Verification items for this drawing (mm, ordinates from the low corner). A direction names the side the tool comes from. Coordinates: 2 decimals unless noted, no trailing zeros. Order: outer loops, then holes, each group sorted by start corner. A loop starts at its lowest first (then second) coordinate and runs counter-clockwise, first axis right, second up. Notation, with made-up numbers: (6, 84.25) -> (47, 84.25) arc R28 cw to (47, 108.25) -> close; hole circle Ø7 at (-39.75, 10.5). An arc over 180 degrees is marked (long way). Answer as CSV lines item,"result". Start each with the question number.
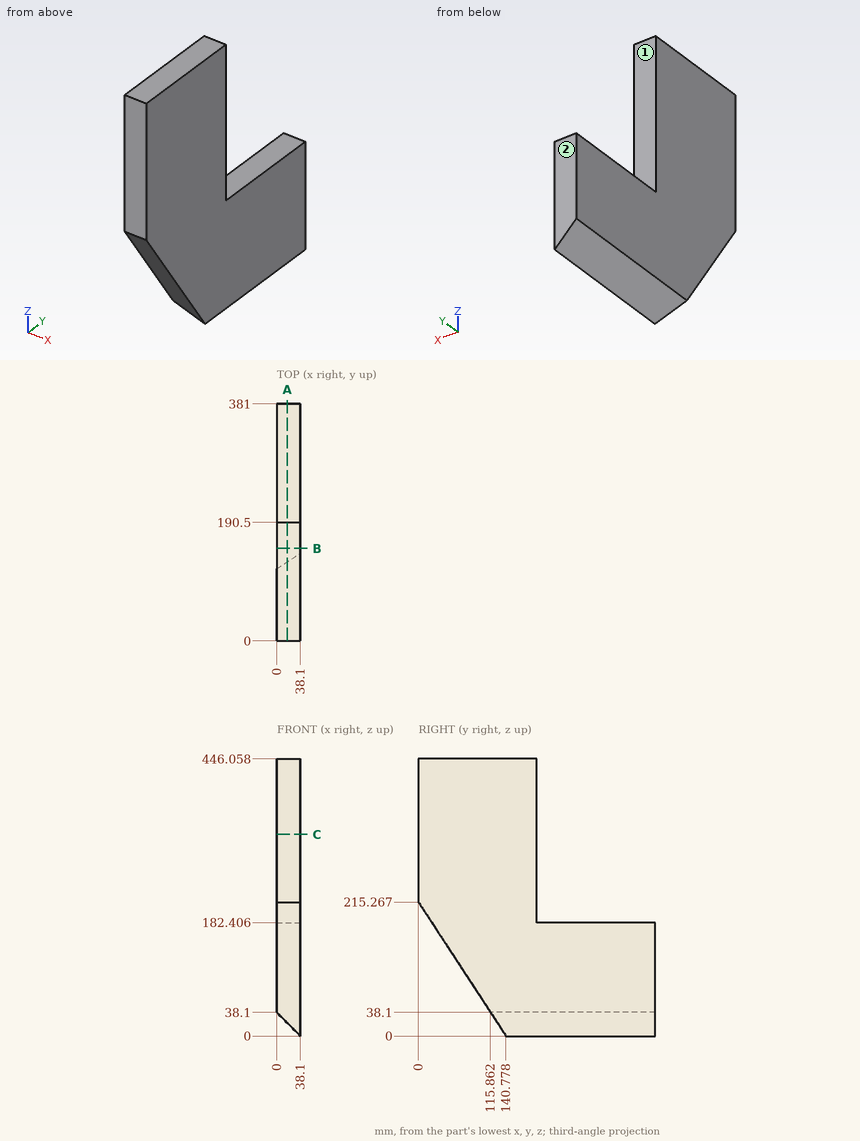
Q1. Go/stop test with flat-tipped pins: pin 1 Ø10 at (x, z) = (6.5, 79) entering from -Y (1 decimal); pin 2 Ø4 at (x, y) = (16, 80) entering from -Z; pin 3 Ø5 at (x, z) = (32.5, 198) entering from +Y. Record where each tip stops, or that it passes through.
Q2. Thickness scan on L1, parallel to Y at x = 33.5, z = 305.5; L2, parallel to Z at x = 20.5, y = 64.5 (1 decimal); L3, parallel to Y at x = 4, z = 109 (1 decimal). Record the ranges inside material, lowest first.
Q3. Sectioned sample at B-B, the plane y = 148.5. Record the cut outline in (x, z), then the cut area to 3 significant figures.
Q4. Sectioned sample at C-C, the plane z = 324.5. Record the cut outline in (x, y), then the cut area to 3 significant figures.
Q5. Access from +Z, -Z, +X, -X, +Y, -Y to the whole of each face (thin tool, end or side, straight path). Record for the marked faces 1 and 2.
Q6. Sectioned sample at A-A, the plane x = 17. Record the cut outline in (y, z) (1 decimal).
Geometry results:
1,pin 1,"stops at y = 85.8"
1,pin 2,"stops at z = 89.88"
1,pin 3,"stops at y = 190.5"
2,L1,"y = 0 to 190.5"
2,L2,"z = 116.6 to 446.1"
2,L3,"y = 69.5 to 381"
3,outline,"(0, 38.1) -> (38.1, 0) -> (38.1, 446.06) -> (0, 446.06) -> close"
3,area,"16,300 mm^2"
4,outline,"(0, 0) -> (38.1, 0) -> (38.1, 190.5) -> (0, 190.5) -> close"
4,area,"7,260 mm^2"
5,face 1,"+Z, +X, -X, +Y"
5,face 2,"+Z, -Z, +X, -X, +Y"
6,outline,"(0, 215.3) -> (127, 21.1) -> (381, 21.1) -> (381, 182.4) -> (190.5, 182.4) -> (190.5, 446.1) -> (0, 446.1) -> close"
